Build history of the part. All positions in model axes, mm. Face numbers are marked on the shaded views. A direction names the side the tool comes from. Round coordinates to 2 decimals unless told otherwise and drop trailing zeros. Write each loop counter-clockwise with the first axis right and the second up, starting at its lowest first coordinate (ties: lowest second). Pieces come first, ordered by that corner, then holes. Notation, with made-up numbers: M 86.5,82 L 99.5,82 A21 ccw 99.5,98 Z; hole C 43,42 d2. An arc over 180 degrees is marked long. Write item = value, one per line. Start each with the question number.
Q1. Pull direction X, two halves, no side cores. Call the marked faces 1, 2, 3 and 4: released by +X, released by -X, zero draft, split by the parting line, or undercut.
Q2. Band-saw the part on A-A on y = 66. Write the cut outline in (x, z).
Q3. Drop flat-ended pins along their axis: P1, Ø6, axis at x = 14, y = 58.5, coming from the -Z side; P2, Ø2.5, axis at y = 75.5, z = 12, coming from the -X side; P3, Ø0.5, axis at x = 2, z = 12.5, coming from the +Y side. Give the stop position or say it passes through.
Q4. Tool access for the marked faces 5 and 6: list every direction of +Z, -Z, +X, -X, +Y, -Y with a clear straight run to the whole face (end or side of a thin tool).
Q5. Probe L1, parallel to X at y = 33.7, z = 12.65; L2, parallel to Y at x = 27.5, z = 11.8; L3, parallel to Y at x = 18, z = 13.5. List the from-to ranges inside material, lowest first.
Q6. Band-saw the part on B-B on y = 86. Write the cut outline in (x, z), plus the area to 3 significant figures.
```python
from build123d import *

# Parameters (mm, degrees)
SKETCH017_W     = 55
SKETCH017_H     = 75.8
PAD012_DEPTH    = 3.6
SKETCH018_W     = 51.76
SKETCH018_H     = 74.18
PAD013_DEPTH    = 5
POCKET004_DEPTH = 7
SKETCH019_R     = 2
PAD014_DEPTH    = 8
SKETCH020_W     = 10
SKETCH020_H     = 2.5
POCKET005_DEPTH = 1
SKETCH021_W     = 10
SKETCH021_H     = 2.5
POCKET006_DEPTH = 1
POCKET007_DEPTH = 2.3
SKETCH023_R     = 1.6
POCKET008_DEPTH = 7.301
CHAMFER010_SIZE = 5
CHAMFER011_SIZE = 2
CHAMFER012_SIZE = 1
CHAMFER013_SIZE = 3
CHAMFER014_SIZE = 0.5
CHAMFER015_SIZE = 1
CHAMFER016_SIZE = 3
CHAMFER017_SIZE = 0.1
CHAMFER018_SIZE = 1


with BuildPart() as part:
    # Sketch017 → Pad012 (new body)
    with BuildSketch(Plane(origin=(55, 28.2, 17.6), x_dir=(-1, 0, 0), z_dir=(0, 0, -1))):
        with Locations((27.5, 37.9)):
            Rectangle(SKETCH017_W, SKETCH017_H)
    extrude(amount=PAD012_DEPTH)

    # Sketch018 → Pad013 (new body)
    with BuildSketch(Plane(origin=(55, 28.2, 14), x_dir=(-1, 0, 0), z_dir=(0, 0, -1))):
        with Locations((27.5, 37.09)):
            Rectangle(SKETCH018_W, SKETCH018_H)
    extrude(amount=PAD013_DEPTH)

    # Sketch002 → Pocket004 (cut)
    with BuildSketch(Plane(origin=(55, 28.2, 9), x_dir=(-1, 0, 0), z_dir=(0, 0, -1))):
        Polygon((18.22, 1.6), (3.22, 1.6), (3.22, 72.58), (51.78, 72.58), (51.78, 1.6), (36.78, 1.6), (36.78, 14.1), (18.22, 14.1), align=None)
    extrude(amount=-POCKET004_DEPTH, mode=Mode.SUBTRACT)

    # Sketch019 → Pad014 (new body)
    with BuildSketch(Plane(origin=(55, 28.2, 16), x_dir=(-1, 0, 0), z_dir=(0, 0, -1))):
        with Locations((10.72, 52.58)):
            Circle(SKETCH019_R)
        with Locations((44.28, 52.58)):
            Circle(SKETCH019_R)
        with Locations((18.22, 18.6)):
            Circle(SKETCH019_R)
        with Locations((36.78, 18.6)):
            Circle(SKETCH019_R)
    extrude(amount=PAD014_DEPTH)

    # Sketch020 → Pocket005 (cut)
    with BuildSketch(Plane(origin=(1.62, 28.2, 17.6), x_dir=(0, 1, 0), z_dir=(-1, 0, 0))):
        with Locations((19, 5.35)):
            Rectangle(SKETCH020_W, SKETCH020_H)
        with Locations((57.5, 5.35)):
            Rectangle(SKETCH020_W, SKETCH020_H)
    extrude(amount=-POCKET005_DEPTH, mode=Mode.SUBTRACT)

    # Sketch021 → Pocket006 (cut)
    with BuildSketch(Plane(origin=(53.38, 28.2, 17.6), x_dir=(0, -1, 0), z_dir=(1, 0, 0))):
        with Locations((-57.5, 5.35)):
            Rectangle(SKETCH021_W, SKETCH021_H)
        with Locations((-19, 5.35)):
            Rectangle(SKETCH021_W, SKETCH021_H)
    extrude(amount=-POCKET006_DEPTH, mode=Mode.SUBTRACT)

    # Sketch022 → Pocket007 (cut)
    with BuildSketch(Plane(origin=(55, 28.2, 17.6), x_dir=(-1, 0, 0), z_dir=(0, 0, 1))):
        with BuildLine():
            Line((22, 0), (33, 0))
            Line((33, 0), (33, -5.500002))
            ThreePointArc((27.500001, -11), (31.389087, -9.389088), (33, -5.500002))
            Line((27.500001, -11), (27.499999, -11))
            ThreePointArc((22, -5.500002), (23.610913, -9.389088), (27.499999, -11))
            Line((22, -5.500002), (22, 0))
        make_face()
    extrude(amount=-POCKET007_DEPTH, mode=Mode.SUBTRACT)

    # Sketch023 → Pocket008 (cut, through all)
    with BuildSketch(Plane(origin=(55, 28.2, 15.3), x_dir=(-1, 0, 0), z_dir=(0, 0, 1))):
        with Locations((27.5, -5.5)):
            Circle(SKETCH023_R)
    extrude(amount=-POCKET008_DEPTH, mode=Mode.SUBTRACT)

    # Chamfer010
    chamfer010_edges = [part.edges().sort_by_distance(p)[0] for p in [
        (36.78, 42.3, 12.5),
        (18.22, 42.3, 12.5),
    ]]
    chamfer(chamfer010_edges, length=CHAMFER010_SIZE)

    # Chamfer011
    chamfer011_edges = [part.edges().sort_by_distance(p)[0] for p in [
        (51.78, 100.78, 12.5),
        (3.22, 100.78, 12.5),
    ]]
    chamfer(chamfer011_edges, length=CHAMFER011_SIZE)

    # Chamfer012
    chamfer012_edges = [part.edges().sort_by_distance(p)[0] for p in [
        (51.78, 64.29, 16),
        (50.78, 99.78, 16),
        (44.28, 29.8, 16),
        (27.5, 100.78, 16),
        (36.78, 33.55, 16),
        (4.22, 99.78, 16),
        (34.28, 39.8, 16),
        (3.22, 64.29, 16),
        (27.5, 42.3, 16),
        (10.72, 29.8, 16),
        (20.72, 39.8, 16),
        (18.22, 33.55, 16),
        (46.28, 80.78, 16),
        (38.78, 46.8, 16),
        (20.22, 46.8, 16),
        (12.72, 80.78, 16),
    ]]
    chamfer(chamfer012_edges, length=CHAMFER012_SIZE)

    # Chamfer013
    chamfer013_edges = [part.edges().sort_by_distance(p)[0] for p in [
        (1.62, 102.38, 11.5),
        (53.38, 102.38, 11.5),
    ]]
    chamfer(chamfer013_edges, length=CHAMFER013_SIZE)

    # Chamfer014
    chamfer014_edges = [part.edges().sort_by_distance(p)[0] for p in [
        (53.38, 63.79, 9),
        (51.88, 100.88, 9),
        (27.5, 28.2, 9),
        (27.5, 102.38, 9),
        (1.62, 63.79, 9),
        (3.12, 100.88, 9),
        (3.22, 64.29, 9),
        (4.22, 99.78, 9),
        (10.72, 29.8, 9),
        (27.5, 100.78, 9),
        (18.22, 33.55, 9),
        (50.78, 99.78, 9),
        (20.72, 39.8, 9),
        (51.78, 64.29, 9),
        (27.5, 42.3, 9),
        (44.28, 29.8, 9),
        (34.28, 39.8, 9),
        (36.78, 33.55, 9),
        (29.1, 33.7, 9),
    ]]
    chamfer(chamfer014_edges, length=CHAMFER014_SIZE)

    # Chamfer015
    chamfer015_edges = [part.edges().sort_by_distance(p)[0] for p in [
        (29.1, 33.7, 15.3),
    ]]
    chamfer(chamfer015_edges, length=CHAMFER015_SIZE)

    # Chamfer016
    chamfer016_edges = [part.edges().sort_by_distance(p)[0] for p in [
        (55, 104, 15.8),
        (0, 104, 15.8),
        (27.5, 104, 17.6),
        (0, 66.1, 17.6),
        (55, 66.1, 17.6),
    ]]
    chamfer(chamfer016_edges, length=CHAMFER016_SIZE)

    # Chamfer017
    chamfer017_edges = [part.edges().sort_by_distance(p)[0] for p in [
        (42.5, 28.2, 17.6),
        (12.5, 28.2, 17.6),
    ]]
    chamfer(chamfer017_edges, length=CHAMFER017_SIZE)

    # Chamfer018
    chamfer018_edges = [part.edges().sort_by_distance(p)[0] for p in [
        (31.389087, 37.589088, 17.6),
    ]]
    chamfer(chamfer018_edges, length=CHAMFER018_SIZE)


solid = part.part
```
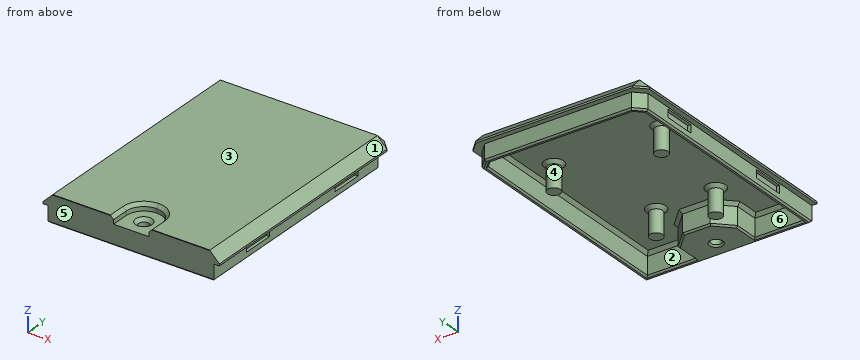
Conclusion:
q1.face_1 = released by +X
q1.face_2 = undercut
q1.face_3 = zero draft
q1.face_4 = undercut
q2.outline = M 0,14 L 1.62,14 L 1.62,9.5 L 2.12,9 L 2.72,9 L 3.22,9.5 L 3.22,15 L 4.22,16 L 50.78,16 L 51.78,15 L 51.78,9.5 L 52.28,9 L 52.88,9 L 53.38,9.5 L 53.38,14 L 55,14 L 55,14.6 L 52,17.6 L 3,17.6 L 0,14.6 Z
q3.P1 = 16
q3.P2 = 1.62
q3.P3 = 100.01
q4.face_5 = +Z, -Z, +X, -X, -Y
q4.face_6 = -Z
q5.L1 = 1.62 to 3.22, 18.22 to 25.9, 29.1 to 36.78, 51.78 to 53.38
q5.L2 = 28.2 to 32.1, 35.3 to 42.3, 100.78 to 102.38
q5.L3 = 28.2 to 29.8, 44.81 to 48.79, 100.78 to 102.38
q6.outline = M 0,14 L 1.62,14 L 1.62,13.5 L 2.62,13.5 L 2.62,11 L 1.62,11 L 1.62,9.5 L 2.12,9 L 2.72,9 L 3.22,9.5 L 3.22,15 L 4.22,16 L 50.78,16 L 51.78,15 L 51.78,9.5 L 52.28,9 L 52.88,9 L 53.38,9.5 L 53.38,11 L 52.38,11 L 52.38,13.5 L 53.38,13.5 L 53.38,14 L 55,14 L 55,14.6 L 52,17.6 L 3,17.6 L 0,14.6 Z
q6.area = 103 mm^2
